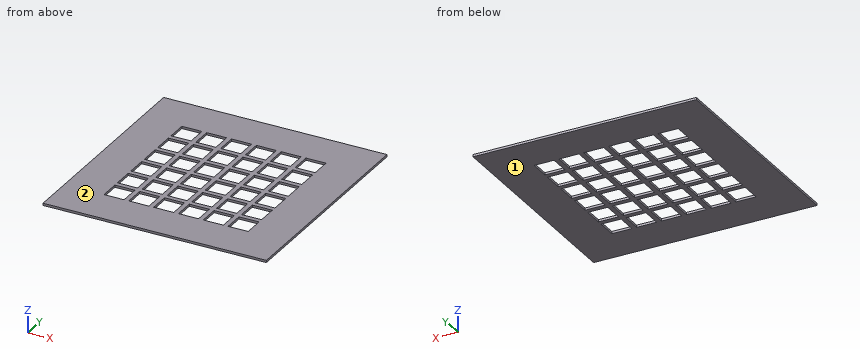
```python
from build123d import *

# Parameters (mm, degrees)
SKETCH050_W                        = 100
SKETCH050_H                        = 100
PAD019_DEPTH                       = 1
SKETCH051_W                        = 9
SKETCH051_H                        = 9
POCKET012_DEPTH                    = 283.850783
SKETCH051_LINEARPATTERN002_2_W     = 9
SKETCH051_LINEARPATTERN002_2_H     = 9
POCKET012_LINEARPATTERN002_2_DEPTH = 283.850783
SKETCH051_LINEARPATTERN002_3_W     = 9
SKETCH051_LINEARPATTERN002_3_H     = 9
POCKET012_LINEARPATTERN002_3_DEPTH = 283.850783
SKETCH051_LINEARPATTERN002_4_W     = 9
SKETCH051_LINEARPATTERN002_4_H     = 9
POCKET012_LINEARPATTERN002_4_DEPTH = 283.850783
SKETCH051_LINEARPATTERN002_5_W     = 9
SKETCH051_LINEARPATTERN002_5_H     = 9
POCKET012_LINEARPATTERN002_5_DEPTH = 283.850783
SKETCH051_LINEARPATTERN002_6_W     = 9
SKETCH051_LINEARPATTERN002_6_H     = 9
POCKET012_LINEARPATTERN002_6_DEPTH = 283.850783
LINEARPATTERN003_COUNT             = 6
LINEARPATTERN003_PITCH             = 11.111111


with BuildPart() as part:
    # Sketch050 → Pad019 (new body)
    with BuildSketch(Plane.XY):
        Rectangle(SKETCH050_W, SKETCH050_H)
    extrude(amount=PAD019_DEPTH)

    # Sketch051 → Pocket012 (cut, through all)
    with BuildSketch(Plane.XY):
        with Locations((-27.777778, 27.777778)):
            Rectangle(SKETCH051_W, SKETCH051_H)
    pocket012 = extrude(amount=POCKET012_DEPTH, mode=Mode.SUBTRACT)

    # Sketch051 LinearPattern002 2 → Pocket012 LinearPattern002 2 (cut, through all)
    with BuildSketch(Plane(origin=(11.111111, 0, 0), x_dir=(1, 0, 0), z_dir=(0, 0, 1))):
        with Locations((-27.777778, 27.777778)):
            Rectangle(SKETCH051_LINEARPATTERN002_2_W, SKETCH051_LINEARPATTERN002_2_H)
    pocket012_linearpattern002_2 = extrude(amount=POCKET012_LINEARPATTERN002_2_DEPTH, mode=Mode.SUBTRACT)

    # Sketch051 LinearPattern002 3 → Pocket012 LinearPattern002 3 (cut, through all)
    with BuildSketch(Plane(origin=(22.222222, 0, 0), x_dir=(1, 0, 0), z_dir=(0, 0, 1))):
        with Locations((-27.777778, 27.777778)):
            Rectangle(SKETCH051_LINEARPATTERN002_3_W, SKETCH051_LINEARPATTERN002_3_H)
    pocket012_linearpattern002_3 = extrude(amount=POCKET012_LINEARPATTERN002_3_DEPTH, mode=Mode.SUBTRACT)

    # Sketch051 LinearPattern002 4 → Pocket012 LinearPattern002 4 (cut, through all)
    with BuildSketch(Plane(origin=(33.333333, 0, 0), x_dir=(1, 0, 0), z_dir=(0, 0, 1))):
        with Locations((-27.777778, 27.777778)):
            Rectangle(SKETCH051_LINEARPATTERN002_4_W, SKETCH051_LINEARPATTERN002_4_H)
    pocket012_linearpattern002_4 = extrude(amount=POCKET012_LINEARPATTERN002_4_DEPTH, mode=Mode.SUBTRACT)

    # Sketch051 LinearPattern002 5 → Pocket012 LinearPattern002 5 (cut, through all)
    with BuildSketch(Plane(origin=(44.444444, 0, 0), x_dir=(1, 0, 0), z_dir=(0, 0, 1))):
        with Locations((-27.777778, 27.777778)):
            Rectangle(SKETCH051_LINEARPATTERN002_5_W, SKETCH051_LINEARPATTERN002_5_H)
    pocket012_linearpattern002_5 = extrude(amount=POCKET012_LINEARPATTERN002_5_DEPTH, mode=Mode.SUBTRACT)

    # Sketch051 LinearPattern002 6 → Pocket012 LinearPattern002 6 (cut, through all)
    with BuildSketch(Plane(origin=(55.555556, 0, 0), x_dir=(1, 0, 0), z_dir=(0, 0, 1))):
        with Locations((-27.777778, 27.777778)):
            Rectangle(SKETCH051_LINEARPATTERN002_6_W, SKETCH051_LINEARPATTERN002_6_H)
    pocket012_linearpattern002_6 = extrude(amount=POCKET012_LINEARPATTERN002_6_DEPTH, mode=Mode.SUBTRACT)

    # LinearPattern003: Pocket012, Pocket012 LinearPattern002 2, Pocket012 LinearPattern002 3, Pocket012 LinearPattern002 4, Pocket012 LinearPattern002 5, Pocket012 LinearPattern002 6 ×6
    with Locations(*[(0, -i * LINEARPATTERN003_PITCH, 0) for i in range(1, LINEARPATTERN003_COUNT)]):
        add(pocket012, mode=Mode.SUBTRACT)
        add(pocket012_linearpattern002_2, mode=Mode.SUBTRACT)
        add(pocket012_linearpattern002_3, mode=Mode.SUBTRACT)
        add(pocket012_linearpattern002_4, mode=Mode.SUBTRACT)
        add(pocket012_linearpattern002_5, mode=Mode.SUBTRACT)
        add(pocket012_linearpattern002_6, mode=Mode.SUBTRACT)


solid = part.part
```
The model under review builds one solid part; all positions refer to its coordinate system, in mm. Face numbers are marked on the shaded views. Round coordinates to 2 decimals unless told otherwise and drop trailing zeros. Loops run counter-clockwise (first coordinate to the right, second up) from the corner with the lowest first, then second, coordinate; pieces in that order, holes last. Notation, with made-up numbers: M 26.25,4.25 L 70.25,4.25 A29 cw 70.25,33.25 Z; hole C 84,18.25 d8. An arc over 180 degrees is marked long. Put each result on its own line as item: value.
Q1. Consider section C-C, the plane z = 0.85. Count the separate pieces of the cut face and the enclosed holes in it, then the cut area to 3 significant figures.
Result set:
separate pieces: 1
enclosed holes: 36
area: 7,080 mm²
Q2. Mouldability with a two-part tool opening along Z and no side actions: class the marked faces 1 and 2 as released by +Z, released by -Z, zero draft, split by the parting line, or undercut.
Result set:
face 1: released by -Z
face 2: released by +Z
Q3. Consider section A-A, the plane y = -25.5. Give the boundary of the cut face in (x, z), then the cut area to 3 significant figures.
Result set:
outline: M -50,0 L -32.28,0 L -32.28,1 L -50,1 Z; M -23.28,0 L -21.17,0 L -21.17,1 L -23.28,1 Z; M -12.17,0 L -10.06,0 L -10.06,1 L -12.17,1 Z; M -1.06,0 L 1.06,0 L 1.06,1 L -1.06,1 Z; M 10.06,0 L 12.17,0 L 12.17,1 L 10.06,1 Z; M 21.17,0 L 23.28,0 L 23.28,1 L 21.17,1 Z; M 32.28,0 L 50,0 L 50,1 L 32.28,1 Z
area: 46.0 mm²
